Autodesk Inventor part; units mm, degrees
ref_plane "YZ Plane" through (0, 0, 0) normal (1, 0, 0) x (0, 1, 0)
ref_plane "XZ Plane" through (0, 0, 0) normal (0, 1, 0) x (-1, 0, 0)
ref_plane "XY Plane" through (0, 0, 0) normal (0, 0, 1) x (1, 0, 0)
sketch "Sketch1" plane through (0, 0, 0) normal (0, 1, 0) x (-1, 0, 0)
  circle A0 centre (0, 0) radius 2.25
  circle A1 centre (0, 0) radius 1.5
  dimension "d0" = 4.5
  dimension "d1" = 3
extrude "Extrusion1" add sketch "Sketch1" against normal blind 10 contours A1
extrude "Extrusion2" add sketch "Sketch1" along normal blind 2 contours A0 | A1
sketch "Sketch2" plane through (0, 2, 0) normal (0, 1, 0) x (1, 0, 0)
  circle A0 centre (0, 0) radius 1.5
  line L0 (-1, -0.5774) -> (-1, 0.5774)
  line L1 (-1, 0.5774) -> (0, 1.1547)
  line L2 (0, 1.1547) -> (1, 0.5774)
  line L3 (1, 0.5774) -> (1, -0.5774)
  line L4 (1, -0.5774) -> (0, -1.1547)
  line L5 (0, -1.1547) -> (-1, -0.5774)
  dimension "d6" = 2
extrude "Extrusion3" cut sketch "Sketch2" against normal blind 1.5 contours L0 L1 L2 L3 L4 L5
equation "\"d0\" = D_"
equation "\"d1\" = M_"
equation "\"d2\" = L_"
equation "\"d4\" = K_"
equation "\"d6\" = S_"
equation "\"d7\" = t_"
equation "\"K_\" = 2"
equation "\"D_\" = 4.5"
equation "\"S_\" = 2"
equation "\"t_\" = 1.5"
equation "\"M_\" = 3"
equation "\"L_\" = 10"
properties part number "M3 x 10" material "Stainless Steel"
Build history of the part. All positions in model axes, mm. A direction names the side the tool comes from. Round coordinates to 2 decimals unless told otherwise and drop trailing zeros. Loops run counter-clockwise (first coordinate to the right, second up) from the corner with the lowest first, then second, coordinate; pieces in that order, holes last. Notation, with made-up numbers: (-32, 75) -> (0, 75) arc R10 cw to (0, 94) -> close; hole circle Ø2 at (54.5, -17). An arc over 180 degrees is marked (long way). One line per item, written item: value. Start each with the question number.
Q1. Probe line 1 along X through (y, z) = (1.5, 0.6); line 2 along Y through (x, z) = (-0.1, 0.85); line 3 along Y through (x, z) = (-0.2, 2). List the from-to ranges inside material, lowest first.
Q2. Two-plate mould, pull along Z, no slides. Class faces 1 (the face through (0, -10, 0)), 2 (the face through (0.29, 0.99, -2.23)), 3 (the face through (0.51, 1.26, 0.86)): released by +Z, released by -Z, zero draft, split by the parting line, or undercut.
Q3. Cut at A-A on z = 0. List the corners of the cut face in (x, y).
Q4. Cut at D-D on x = 1.2. List the corners of the cut face in (y, z), plus the area to 3 significant figures.
Q5. Cut at B-B on x = -0.8. List the corners of the cut face in (y, z), plus the area to 3 significant figures.
Q6. 3-axis set-ups, long thin cutter, end or side, ignore diameter. For faces 4 (the face through (-0.51, 1.26, -0.86)), 5 (the face through (1.5, -4.93, 0.07)), 6 (the face through (1, 2, -1)): which of +Z, -Z, +X, -X, +Y, -Y reach the whole face in a straight line?
Q7. Drop flat-ended pins along their axis: pin 1 Ø1.5 at (y, z) = (-8.5, -1) entering from -X; pin 2 Ø2 at (y, z) = (-3.5, 1.5) entering from +X; pin 3 Ø0.6 at (y, z) = (1.5, 0.5) entering from +X. Give the stop position or say it passes through.
Q8. Cut at C-C on y = -6.5. List the corners of the cut face in (x, z).
Computed:
1. line 1: -2.17 to -0.96, 0.96 to 2.17
1. line 2: -10 to 0.5
1. line 3: 0 to 2
2. face 1: zero draft
2. face 2: split by the parting line
2. face 3: undercut
3. outline: (-2.25, 0) -> (-1.5, 0) -> (-1.5, -10) -> (1.5, -10) -> (1.5, 0) -> (2.25, 0) -> (2.25, 2) -> (1, 2) -> (1, 0.5) -> (-1, 0.5) -> (-1, 2) -> (-2.25, 2) -> close
4. outline: (-10, -0.9) -> (0, -0.9) -> (0, -1.9) -> (2, -1.9) -> (2, 1.9) -> (0, 1.9) -> (0, 0.9) -> (-10, 0.9) -> close
4. area: 25.6 mm²
5. outline: (-10, -1.27) -> (0, -1.27) -> (0, -2.1) -> (2, -2.1) -> (2, -0.69) -> (0.5, -0.69) -> (0.5, 0.69) -> (2, 0.69) -> (2, 2.1) -> (0, 2.1) -> (0, 1.27) -> (-10, 1.27) -> close
5. area: 31.7 mm²
6. face 4: +Y
6. face 5: -Y
6. face 6: +Z, -Z, +X, -X, +Y
7. pin 1: x = -1.48
7. pin 2: x = 1.41
7. pin 3: x = 2.24
8. outline: circle Ø3 at (0, 0)
